```python
from build123d import *

# Parameters (mm, degrees)
SKETCH1_W           = 40
SKETCH1_H           = 40
BOSS_EXTRUDE1_DEPTH = 10
SKETCH2_R           = 1.32
CUT_EXTRUDE2_DEPTH  = 5
SKETCH5_R           = 3
CUT_EXTRUDE3_DEPTH  = 5


with BuildPart() as part:
    # Sketch1 → Boss-Extrude1 (new body)
    with BuildSketch(Plane.XY):
        with Locations((-20, -20)):
            Rectangle(SKETCH1_W, SKETCH1_H)
    extrude(amount=BOSS_EXTRUDE1_DEPTH)

    # Sketch2 → Cut-Extrude2 (cut)
    with BuildSketch(Plane.XY):
        with Locations((-35.87, -35.875)):
            Circle(SKETCH2_R)
        with Locations((-4.12, -35.875)):
            Circle(SKETCH2_R)
        with Locations((-4.12, -4.125)):
            Circle(SKETCH2_R)
        with Locations((-35.87, -4.125)):
            Circle(SKETCH2_R)
    extrude(amount=CUT_EXTRUDE2_DEPTH, mode=Mode.SUBTRACT)

    # Sketch5 → Cut-Extrude3 (cut)
    with BuildSketch(Plane.XY.offset(10)):
        with Locations((-32.7, -7.3)):
            Circle(SKETCH5_R)
        with Locations((-7.3, -7.3)):
            Circle(SKETCH5_R)
        with Locations((-7.3, -32.7)):
            Circle(SKETCH5_R)
        with Locations((-32.7, -32.7)):
            Circle(SKETCH5_R)
    extrude(amount=-CUT_EXTRUDE3_DEPTH, mode=Mode.SUBTRACT)


solid = part.part
```
Input: part model. Units: mm. Frame: model coordinates. A direction names the side the tool comes from. Coordinates: 2 decimals unless noted, no trailing zeros. Write each loop counter-clockwise with the first axis right and the second up, starting at its lowest first coordinate (ties: lowest second). Pieces come first, ordered by that corner, then holes. Notation, with made-up numbers: (9.25, 5) - (66.25, 5) arc R19 cw to (66.25, 39) - close; hole circle Ø8 at (79, 46.25). An arc over 180 degrees is marked (long way). Put each result on its own line as item: value. Start each with the question number.
1) Reachability of faces 4 (the face through (-36, -36, 5)), 5 (the face through (-33, -33, 5)), 6 (the face through (-20, -20, 0)) from +Z, -Z, +X, -X, +Y, -Y: full face, straight path, thin tool, end or side. Return the list, or none.
2) Ray query, L1, parallel to Y at x = -32.7, z = 7.8; L2, parallel to Y at x = -4.12, z = 1.9 (3 decimals); L3, parallel to X at y = -33, z = 5.25. Return the intervals inside material, ascending.
3) Contact query for flat-ended pins moving along their axis: pin 1 (2.5 mm diameter, centred on x = -4.12, y = -4.125, fed in from -Z); pin 2 (1.8 mm diameter, centred on x = -8, y = -32, fed in from +Z). Output: stop coordinate, or through.
4) Cut plane A-A (z = 8). Return the cut outline in (x, y), plus the area to 3 significant figures.
5) Mould query, pull axis X, two halves, no side actions, for faces 1 (the face through (0, -20, 5)), 2 (the face through (-7.691, -29.726, 7.535)), 3 (the face through (-20, -20, 10)). Classes: pulls with the +X half, pulls with the -X half, needs draft (parallel to the pull), parting line crosses it, or undercut.
6) Cut plane B-B (x = -7.3). Return the cut outline in (y, z), plus the area to 3 significant figures.
Resolved:
1. face 4: -Z
1. face 5: +Z
1. face 6: -Z, +X, -X, +Y, -Y
2. L1: y = -40 to -35.7, -29.7 to -10.3, -4.3 to 0
2. L2: y = -40 to -37.195, -34.555 to -5.445, -2.805 to 0
2. L3: x = -40 to -35.68, -29.72 to -10.28, -4.32 to 0
3. pin 1: stops at z = 5
3. pin 2: stops at z = 5
4. outline: (-40, -40) - (0, -40) - (0, 0) - (-40, 0) - close; hole circle Ø6 at (-32.7, -32.7); hole circle Ø6 at (-32.7, -7.3); hole circle Ø6 at (-7.3, -32.7); hole circle Ø6 at (-7.3, -7.3)
4. area: 1,490 mm2
5. face 1: pulls with the +X half
5. face 2: undercut
5. face 3: needs draft
6. outline: (-40, 0) - (0, 0) - (0, 10) - (-4.3, 10) - (-4.3, 5) - (-10.3, 5) - (-10.3, 10) - (-29.7, 10) - (-29.7, 5) - (-35.7, 5) - (-35.7, 10) - (-40, 10) - close
6. area: 340 mm2
